Answer from the drawing. Dimensions are ordinates in mm from the lowest x, y and z of the part. Give positions to 0.01 mm unless a question says otherwise; leave off trailing zeros. Loops run counter-clockwise (first coordinate to the right, second up) from the corner with the lowest first, then second, coordinate; pieces in that order, holes last.
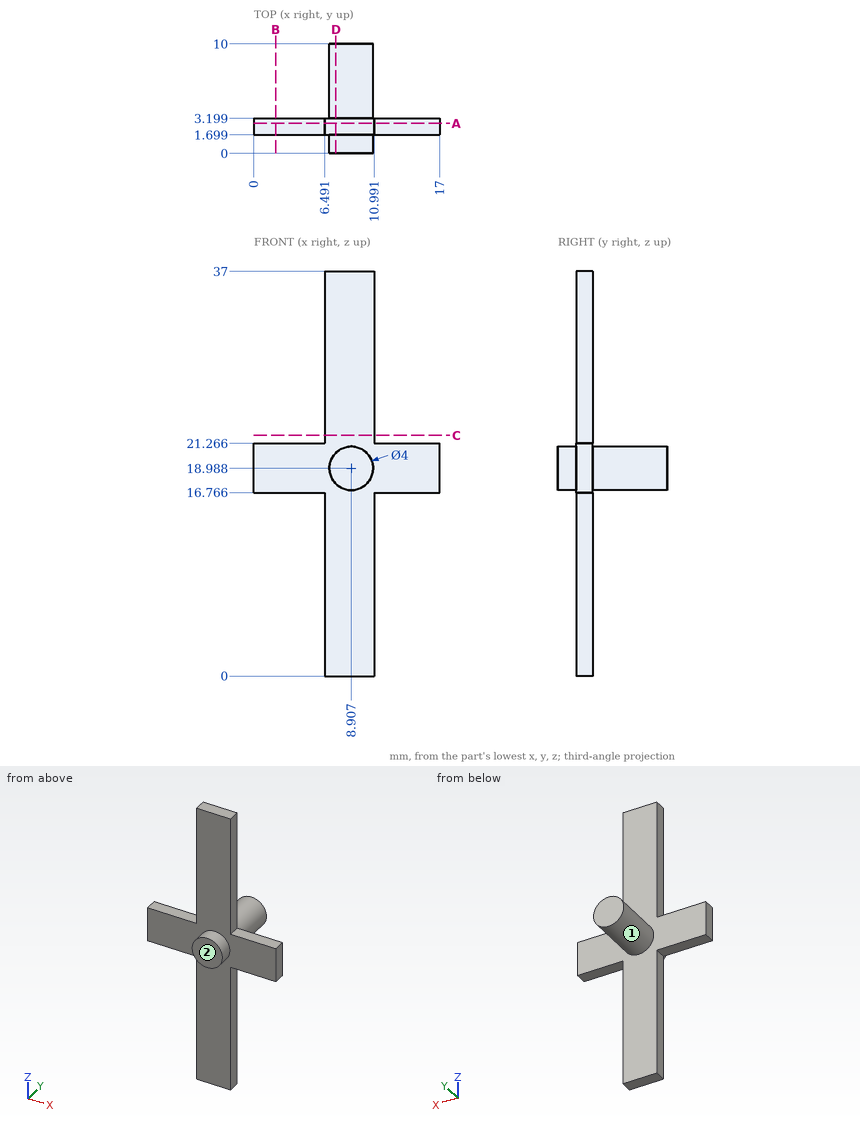
Item 1: Find section A-A, the plane y = 2.75. Write down the section's boundary in (x, z) (1 decimal).
Item 2: Determine the mould class of the marked faces 1 and 2 for opening direction Z: released by +Z, released by -Z, zero draft, split by the parting line, or undercut.
Item 3: Find section D-D, the plane x = 7.5. Write down the section's boundary in (y, z) (1 decimal).
Item 4: Find section B-B, the plane x = 2. Write down the section's boundary in (y, z) (1 decimal).
Item 5: Flat-ended cylindrical pins translate along their axes: pin 1 Ø6 at (y, z) = (4.5, 32.5) entering from -X; pin 2 Ø1.2 at (x, y) = (15, 2.5) entering from +Z; pin 3 Ø1.2 at (x, y) = (3.5, 2.5) entering from -Z. Find the tip coordinate at first contact, or state that the pin passes through.
Item 6: Consider line 1 (Z direction, x = 9, y = 4.5) (1 decimal); line 2 (Y direction, x = 1, z = 19); line 3 (X direction, y = 2.25, z = 2). Determine where each line is inside the solid, lowest interval first.
Item 7: Find section C-C, the plane z = 22. Write down the section's boundary in (x, y).
Ans:
1. outline: (0, 16.8) - (6.5, 16.8) - (6.5, 0) - (11, 0) - (11, 16.8) - (17, 16.8) - (17, 21.3) - (11, 21.3) - (11, 37) - (6.5, 37) - (6.5, 21.3) - (0, 21.3) - close
2. face 1: split by the parting line
2. face 2: zero draft
3. outline: (0, 17.6) - (1.7, 17.6) - (1.7, 0) - (3.2, 0) - (3.2, 17.6) - (10, 17.6) - (10, 20.4) - (3.2, 20.4) - (3.2, 37) - (1.7, 37) - (1.7, 20.4) - (0, 20.4) - close
4. outline: (1.7, 16.8) - (3.2, 16.8) - (3.2, 21.3) - (1.7, 21.3) - close
5. pin 1: stops at x = 6.49
5. pin 2: stops at z = 21.27
5. pin 3: stops at z = 16.77
6. line 1: z = 17 to 21
6. line 2: y = 1.7 to 3.2
6. line 3: x = 6.49 to 10.99
7. outline: (6.49, 1.7) - (10.99, 1.7) - (10.99, 3.2) - (6.49, 3.2) - close
